CAD build for the part. Positions are in the model's coordinates, mm. A direction names the side the tool comes from. Round coordinates to 2 decimals unless told otherwise and drop trailing zeros. Write each loop counter-clockwise with the first axis right and the second up, starting at its lowest first coordinate (ties: lowest second). Pieces come first, ordered by that corner, then holes. Notation, with made-up numbers: (5, -1.75) - (35, -1.75) arc R26 cw to (35, 34.25) - close; hole circle Ø2 at (-6.5, -23.5). An arc over 180 degrees is marked (long way). Put each result on its own line as item: value. Start each with the question number.
Item 1: 3-axis set-ups, long thin cutter, end or side, ignore diameter. For faces 1 (the flat face through (-1.616, -6, 0)), 2 (the flat face through (-20, -6, -7.75)), 3 (the flat face through (20, -6, 7.75)), 4 (the cylindrical face through (-18.73, -11.51, 0.45)): which of +Z, -Z, +X, -X, +Y, -Y reach the whole face in a straight line?
Item 2: Cut at B-B (z = 0). Count the separate pieces of the cut face and the enclosed holes in it, and give its area (3 significant figures).
Item 3: Cut at C-C (x = -31.25). Give the cut face in (y, z), and give its area (3 significant figures).
Item 4: Pin check, flat tips, straight feed: pin 1 Ø5 at (x, y) = (11.5, -10) entering from +Z; pin 2 Ø7.5 at (y, z) = (-7, -1.5) entering from -X; pin 3 Ø6 at (x, y) = (-19, -3.5) entering from -Z; pin 4 Ø3.5 at (x, z) = (-20.16, 0) entering from -Y. Stop position of each tip, or through.
Item 5: Drill centre lines: line 1 (X direction, y = -0.75, z = 3.5); line 2 (X direction, y = -5, z = -0.25); line 3 (X direction, y = -5.5, z = -6). Where is each one in solid material? Low to high. Write a range as from..to.
Item 6: Mould opens along X. For faces 5 (the flat face through (24.25, -6, 0)), 6 (the cylindrical face through (18.66, -11.51, 2.85)), 7 (the flat face through (16.25, -6, 0)), 8 (the flat face through (-20, -6, 7.75)) say: released by +X, released by -X, zero draft, split by the parting line, or undercut.
Item 7: Cut at A-A (y = -5). Give the cut face in (x, z).
Item 8: Cut at D-D (x = -10). Give the cut face in (y, z).
```python
from build123d import *

# Parameters (mm, degrees)
F0_W     = 72.5
F0_H     = 20
F1_DEPTH = 2
F2_R     = 1.5
F3_DEPTH = 2
F4_W     = 8
F4_H     = 15.5
F4_W_2   = 13.217593
F4_H_2   = 9.198598
F4_R     = 2.5
F5_DEPTH = 12
F6_R     = 1.5
F7_DEPTH = 1


with BuildPart() as f1:
    # F0 (on Front) → F1 (new body)
    with BuildSketch(Plane.XZ):
        Rectangle(F0_W, F0_H)
    extrude(amount=-F1_DEPTH)

    # F2 (on face) → F3 (cut, through all)
    with BuildSketch(Plane.XZ):
        with Locations((-31.25, 0)):
            Circle(F2_R)
        with Locations((31.25, 0)):
            Circle(F2_R)
    extrude(amount=-F3_DEPTH, mode=Mode.SUBTRACT)

    # F4 (on face) → F5 (join)
    with BuildSketch(Plane.XZ):
        with Locations((-20.25, 0)):
            Rectangle(F4_W, F4_H)
        with Locations((20.25, 0)):
            Rectangle(F4_W, F4_H)
        with Locations((-8.224997, 0)):
            Rectangle(F4_W_2, F4_H_2)
        with Locations((9.300935, 0)):
            Circle(F4_R)
    extrude(amount=F5_DEPTH)

    # F6 (on face) → F7 (cut)
    with BuildSketch(Plane.XZ.offset(12)):
        with Locations((-20.159207, 4.766709)):
            Circle(F6_R)
        with Locations((-20.159207, 0)):
            Circle(F6_R)
        with Locations((-20.159207, -4.965322)):
            Circle(F6_R)
        with Locations((20.159205, 2.78058)):
            Circle(F6_R)
        with Locations((20.159205, -2.184742)):
            Circle(F6_R)
    extrude(amount=-F7_DEPTH, mode=Mode.SUBTRACT)


solid = f1.part
```
Output values:
1. face 1: +Z, -Z, -Y
1. face 2: -Z, +X, -X, -Y
1. face 3: +Z, +X, -X, -Y
1. face 4: -Y
2. separate pieces: 3
2. enclosed holes: 0
2. area: 541 mm2
3. outline: (0, -10) - (2, -10) - (2, -1.5) - (0, -1.5) - close; (0, 1.5) - (2, 1.5) - (2, 10) - (0, 10) - close
3. area: 34.0 mm2
4. pin 1: z = 2.5
4. pin 2: x = -24.25
4. pin 3: z = -7.75
4. pin 4: y = -12
5. line 1: -24.25..-16.25, -14.83..-1.62, 16.25..24.25
5. line 2: -24.25..-16.25, -14.83..-1.62, 6.81..11.79, 16.25..24.25
5. line 3: -24.25..-16.25, 16.25..24.25
6. face 5: released by +X
6. face 6: undercut
6. face 7: undercut
6. face 8: zero draft
7. outline: (-24.25, -7.75) - (-16.25, -7.75) - (-16.25, 7.75) - (-24.25, 7.75) - close; (-14.83, -4.6) - (-1.62, -4.6) - (-1.62, 4.6) - (-14.83, 4.6) - close; circle Ø5 at (9.3, 0); (16.25, -7.75) - (24.25, -7.75) - (24.25, 7.75) - (16.25, 7.75) - close
8. outline: (-12, -4.6) - (0, -4.6) - (0, -10) - (2, -10) - (2, 10) - (0, 10) - (0, 4.6) - (-12, 4.6) - close
